from build123d import *

# Parameters (mm, degrees)
F1_DEPTH = 63.5
F2_DEPTH = 7.9375
F0_W     = 25.248305
F0_H     = 19.05
F3_DEPTH = 25.4
F5_R     = 6.35


with BuildPart() as f1:
    # F0 (on Front) → F1 (new body, symmetric)
    with BuildSketch(Plane.XZ):
        Polygon((28.575, 9.525), (-47.625, 9.525), (-47.625, -9.525), (47.625, -9.525), (47.625, 9.525), align=None)
    extrude(amount=F1_DEPTH, both=True)

    # F0 (on Front) → F2 (join, symmetric)
    with BuildSketch(Plane.XZ):
        with BuildLine():
            add(Edge.make_bspline(
                [(-47.625, 9.525), (-47.625, 33.3817), (0, 61.9252), (63.5, 61.9252)],
                knots=[0, 0, 0, 0, 122.859866, 122.859866, 122.859866, 122.859866], degree=3))
            Line((-47.625, 9.525), (28.575, 9.525))
            Line((28.575, 9.525), (28.575, 27.0002))
            ThreePointArc((28.575, 27.0002), (38.804296, 51.695904), (63.5, 61.9252))
        make_face()
    extrude(amount=F2_DEPTH, both=True)

    # F0 (on Front) → F3 (join, symmetric)
    with BuildSketch(Plane.XZ):
        with BuildLine():
            Line((28.575, 27.0002), (28.575, 9.525))
            Line((28.575, 9.525), (47.625, 9.525))
            Line((47.625, 9.525), (47.625, 27.0002))
            ThreePointArc((47.625, 27.0002), (52.27468, 38.22552), (63.5, 42.8752))
            Line((63.5, 42.8752), (66.675, 42.8752))
            Line((66.675, 42.8752), (66.675, 61.9252))
            Line((66.675, 61.9252), (63.5, 61.9252))
            ThreePointArc((63.5, 61.9252), (38.804296, 51.695904), (28.575, 27.0002))
        make_face()
        with Locations((79.299152, 52.4002)):
            Rectangle(F0_W, F0_H)
    extrude(amount=F3_DEPTH, both=True)

    # F0 (on Front) → F4 (revolve)
    with BuildSketch(Plane.XZ):
        Polygon((91.923305, 66.675), (91.923305, 61.9252), (91.923305, 42.8752), (91.923305, 38.1), (117.475, 38.1), (117.475, 66.675), align=None)
    revolve(axis=Axis((91.923305, 0, 52.3875), (0, 0, -1)))

    # F5
    f5_edges = [f1.edges().sort_by_distance(p)[0] for p in [
        (47.625, -63.5, 0),
        (-47.625, -63.5, 0),
        (-47.625, 63.5, 0),
        (47.625, 63.5, 0),
    ]]
    fillet(f5_edges, radius=F5_R)


solid = f1.part
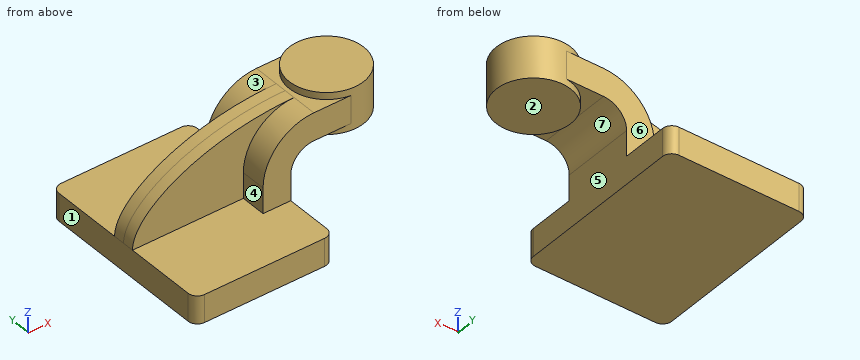
The listing builds one solid part. Answer for the finished solid, in the listing's coordinates (mm). Face numbers are marked on the shaded views. A direction names the side the tool comes from. Give positions to 0.01 mm unless a question says otherwise; leave off trailing zeros. Loops run counter-clockwise (first coordinate to the right, second up) from the corner with the lowest first, then second, coordinate; pieces in that order, holes last. Notation, with made-up numbers: M 24,-38.75 L 68,-38.75 A20 ccw 68,-14.75 Z; hole C 28.25,62 d10. An arc over 180 degrees is marked long. Answer as CSV lines item,"result".
Item 1: Straight lines are drawn through the part: line 1 along Z through (x, y) = (63, 18); line 2 along X through (y, z) = (-18, 7) (3 decimals); line 3 along Z through (x, y) = (-4.5, 16) (3 decimals). For each, find the intervals that lie inside material, in ascending order. Write a range as [from, to].
Values follow:
line 1,"z = [42.87, 61.92]"
line 2,"x = [-47.625, 47.625]"
line 3,"z = [-9.525, 9.525]"
Item 2: Which of the six approach directions +Z, -Z, +X, -X, +Y, -Y give full straight-line access (tool end or side, diameter ignored) to the marked faces 1, 2, 3 and 4?
Values follow:
face 1,"+Z, -Z, -X, +Y, -Y"
face 2,"-Z, +X, +Y, -Y"
face 3,"+Z, -X, +Y"
face 4,"+Z, -X, -Y"
Item 3: The part is cut by section A-A (z = 4.5). Give the vertices of the cut face in (x, y) (3 decimals), and give its area (3 significant figures).
Values follow:
outline,"M -47.625,-57.15 A6.35 ccw -41.275,-63.5 L 41.275,-63.5 A6.35 ccw 47.625,-57.15 L 47.625,57.15 A6.35 ccw 41.275,63.5 L -41.275,63.5 A6.35 ccw -47.625,57.15 Z"
area,"12,100 mm^2"
Item 4: The mould has two halves that part along X. Classify the marked faces 5, 6 and 7: released by +X, released by -X, zero draft, split by the parting line, or undercut.
Values follow:
face 5,"released by +X"
face 6,"zero draft"
face 7,"undercut"
Item 5: Given pin 1 Ø5 at (x, z) = (3, 45) entering from -Y; pin 2 Ø20.5 at (x, y) = (73, -4.5) entering from -Z; pin 3 Ø18.5 at (y, z) = (-0.5, 3.5) entering from +X (3 decimals), each flat-ended and moving along its own axis, determine where each tip first touches the part or whether it passes through.
Values follow:
pin 1,"stops at y = -7.94"
pin 2,"stops at z = 38.1"
pin 3,"stops at x = 47.625"
Item 6: The part is cut by section B-B (y = 29.5). Give the vertices of the cut face in (x, z) (3 decimals).
Values follow:
outline,"M -47.625,-9.525 L 47.625,-9.525 L 47.625,9.525 L -47.625,9.525 Z"
